Can you work these out from the model? Positions are in its coordinate system, mm. A direction names the side the tool comes from. Round coordinates to 2 decimals unless told otherwise and drop trailing zeros. Loops run counter-clockwise (first coordinate to the right, second up) from the corner with the lowest first, then second, coordinate; pieces in that order, holes last. Notation, with made-up numbers: (13.5, 61) -> (46.5, 61) arc R24 cw to (46.5, 86) -> close; hole circle Ø8 at (-5.5, 9). An arc over 180 degrees is marked (long way). Use a Markdown table: item, result.
from build123d import *

# Parameters (mm, degrees)
SKETCH1_R           = 16.4703125
BOSS_EXTRUDE1_DEPTH = 68.659375
SKETCH2_R           = 16.4703125
BOSS_EXTRUDE2_DEPTH = 34.3296875
SKETCH3_R           = 11.7078125
CUT_EXTRUDE1_DEPTH  = 34.3296875
SKETCH4_R           = 13.2953125
CUT_EXTRUDE2_DEPTH  = 25.796875
SKETCH5_R           = 11.7078125
CUT_EXTRUDE3_DEPTH  = 79.51056243


with BuildPart() as part:
    # Sketch1 → Boss-Extrude1 (new body)
    with BuildSketch(Plane.XY):
        Circle(SKETCH1_R)
    extrude(amount=BOSS_EXTRUDE1_DEPTH)

    # Sketch2 → Boss-Extrude2 (add)
    with BuildSketch(Plane(origin=(0, 0, 0), x_dir=(0, 0, -1), z_dir=(1, 0, 0))):
        with Locations((-34.3296875, 0)):
            Circle(SKETCH2_R)
    extrude(amount=BOSS_EXTRUDE2_DEPTH)

    # Sketch3 → Cut-Extrude1 (cut)
    with BuildSketch(Plane(origin=(34.3296875, 0, 0), x_dir=(0, 0, -1), z_dir=(1, 0, 0))):
        with Locations((-34.3296875, 0)):
            Circle(SKETCH3_R)
    extrude(amount=-CUT_EXTRUDE1_DEPTH, mode=Mode.SUBTRACT)

    # Sketch4 → Cut-Extrude2 (cut)
    with BuildSketch(Plane(origin=(34.3296875, 0, 0), x_dir=(0, 0, -1), z_dir=(1, 0, 0))):
        with Locations((-34.647030574, 0)):
            Circle(SKETCH4_R)
    extrude(amount=-CUT_EXTRUDE2_DEPTH, mode=Mode.SUBTRACT)

    # Sketch5 → Cut-Extrude3 (cut, through all)
    with BuildSketch(Plane(origin=(0, 0, 0), x_dir=(-1, 0, 0), z_dir=(0, 0, -1))):
        Circle(SKETCH5_R)
    extrude(amount=-CUT_EXTRUDE3_DEPTH, mode=Mode.SUBTRACT)


solid = part.part
1. I want a section at A-A (y = 0). Please give me the cut outline in (x, z), plus the area to 3 significant figures.
Answer sheet:
| item | result |
|---|---|
| outline | (-16.47, 0) -> (-11.71, 0) -> (-11.71, 68.66) -> (-16.47, 68.66) -> close; (11.71, 0) -> (16.47, 0) -> (16.47, 17.86) -> (34.33, 17.86) -> (34.33, 21.35) -> (11.71, 21.35) -> close; (11.71, 47.94) -> (34.33, 47.94) -> (34.33, 50.8) -> (16.47, 50.8) -> (16.47, 68.66) -> (11.71, 68.66) -> close |
| area | 641 mm² |
2. Will these pins go through, and if not, where does the flat tip stop? pin 1 Ø6 at (x, z) = (24, 45.5) entering from +Y; pin 2 Ø6 at (x, y) = (20, 9) entering from -Z; pin 3 Ø1 at (x, z) = (6, 13.5) entering from -Y.
Answer sheet:
| item | result |
|---|---|
| pin 1 | stops at y = 14.3 |
| pin 2 | stops at z = 18.99 |
| pin 3 | stops at y = -15.52 |
3. I want a section at B-B (x = 12.5). Please give me the cut outline in (y, z), plus the area to 3 significant figures.
Answer sheet:
| item | result |
|---|---|
| outline | (-10.72, 0) -> (10.72, 0) -> (10.72, 21.83) arc R16.47 ccw to (10.72, 46.83) -> (10.72, 68.66) -> (-10.72, 68.66) -> (-10.72, 46.83) arc R16.47 ccw to (-10.72, 21.83) -> close; hole circle Ø26.59 at (0, 34.65) |
| area | 1,120 mm² |
4. Which directions (+Z, -Z, +X, -X, +Y, -Y) give clear straight access to the entire face, cutting with the end or side of a thin tool? Please do faces 5 (the flat face through (8.533, 12, 35)), 6 (the cylindrical face through (-16.454, 0.724, 33.849)), 7 (the cylindrical face through (-11.167, 3.517, 33.849)).
Answer sheet:
| item | result |
|---|---|
| face 5 | +X |
| face 6 | none |
| face 7 | +Z, -Z |
5. I want a section at D-D (z = 42). Please give me the cut outline in (x, y), plus the area to 3 significant figures.
Answer sheet:
| item | result |
|---|---|
| outline | (7.67, -14.58) -> (34.33, -14.58) -> (34.33, -11.08) -> (8.53, -11.08) -> (8.53, -8.85) -> (7.67, -8.85) arc R11.71 cw (long way) to (7.67, 8.85) -> (8.53, 8.85) -> (8.53, 11.08) -> (34.33, 11.08) -> (34.33, 14.58) -> (7.67, 14.58) arc R16.47 ccw (long way) to start |
| area | 479 mm² |
6. If we mould it in two halves opening along Z, with no side actions, what happens to faces 1 (the flat face through (8.533, -12, 35)), 2 (the flat face through (-3.9, 11.2, 68.659)), 3 (the flat face through (34.33, -5, 22)), 4 (the flat face through (-3.9, 11.2, 0))? For each: +Z half, -Z half, draft (parallel to the pull), parting line (faces both ways), or undercut.
Answer sheet:
| item | result |
|---|---|
| face 1 | undercut |
| face 2 | +Z half |
| face 3 | draft |
| face 4 | -Z half |
7. I need wall thicknesses on line 1 (Y direction, x = 0, z = 43); line 2 (Y direction, x = 18.5, z = 35); line 3 (Z direction, x = 15.5, y = 0). Which ranges of each line are inside material? Lowest first, please.
Answer sheet:
| item | result |
|---|---|
| line 1 | y = -16.47 to -11.71, 11.71 to 16.47 |
| line 2 | y = -16.46 to -13.29, 13.29 to 16.46 |
| line 3 | z = 0 to 21.35, 47.94 to 68.66 |
8. I want a section at C-C (y = 7). Please give me the cut outline in (x, z), plus the area to 3 significant figures.
Answer sheet:
| item | result |
|---|---|
| outline | (-14.91, 0) -> (-9.38, 0) -> (-9.38, 68.66) -> (-14.91, 68.66) -> close; (9.38, 0) -> (14.91, 0) -> (14.91, 19.42) -> (34.33, 19.42) -> (34.33, 23.34) -> (9.38, 23.34) -> close; (9.38, 45.95) -> (34.33, 45.95) -> (34.33, 49.24) -> (14.91, 49.24) -> (14.91, 68.66) -> (9.38, 68.66) -> close |
| area | 774 mm² |
